Autodesk Inventor part; units mm, degrees
ref_plane "YZ Plane" through (0, 0, 0) normal (1, 0, 0) x (0, 1, 0)
ref_plane "XZ Plane" through (0, 0, 0) normal (0, 1, 0) x (-1, 0, 0)
ref_plane "XY Plane" through (0, 0, 0) normal (0, 0, 1) x (1, 0, 0)
sketch "Sketch1" plane through (0, 0, 0) normal (0, 0, 1) x (1, 0, 0)
  arc A0 (14.2748, -15.875) -> (15.875, -14.2748) centre (14.2748, -14.2748) ccw
  line L0 (15.875, -14.2748) -> (15.875, 14.2748)
  arc A1 (15.875, 14.2748) -> (14.2748, 15.875) centre (14.2748, 14.2748) ccw
  arc A2 (-14.2748, 15.875) -> (-15.875, 14.2748) centre (-14.2748, 14.2748) ccw
  line L1 (-15.875, 14.2748) -> (-15.875, -14.2748)
  arc A3 (-15.875, -14.2748) -> (-14.2748, -15.875) centre (-14.2748, -14.2748) ccw
  line L2 (-14.2748, -15.875) -> (14.2748, -15.875)
  line L3 (14.2748, 15.875) -> (-14.2748, 15.875)
  line L4 (-15.875, -19.05) -> (56.769, -19.05)
  line L5 (56.769, -19.05) -> (57.15, -18.669)
  line L6 (57.15, -18.669) -> (57.15, -16.256)
  line L7 (57.15, -16.256) -> (56.769, -15.875)
  line L8 (56.769, -15.875) -> (20.6502, -15.875)
  arc A4 (19.05, -14.2748) -> (20.6502, -15.875) centre (20.6502, -14.2748) ccw
  line L9 (19.05, -14.2748) -> (19.05, 15.875)
  arc A5 (19.05, 15.875) -> (15.875, 19.05) centre (15.875, 15.875) ccw
  line L10 (15.875, 19.05) -> (-15.875, 19.05)
  arc A6 (-15.875, 19.05) -> (-19.05, 15.875) centre (-15.875, 15.875) ccw
  line L11 (-19.05, 15.875) -> (-19.05, -15.875)
  arc A7 (-19.05, -15.875) -> (-15.875, -19.05) centre (-15.875, -15.875) ccw
  point P0 (0, 0)
extrude "Extrusion1" add sketch "Sketch1" against normal blind 304.8
hole "Hole1" at (0, 19.05, -19.05) direction (0, -1, 0) diameter 8.3312 end through all
hole "Hole2" at (-19.05, 0, -19.05) direction (1, 0, 0) diameter 8.3312 end through all
pattern_linear "Rectangular Pattern1" count 200 spacing 38.1 along (0, 0, -1) of "Hole1", "Hole2"
properties part number "9706"
Verification items for the finished model (mm, model axes). A direction names the side the tool comes from. Give positions to 0.01 mm unless a question says otherwise; leave off trailing zeros. Order: outer loops, then holes, each group sorted by start corner. A loop starts at its lowest first (then second) coordinate and runs counter-clockwise, first axis right, second up. Notation, with made-up numbers: M 10.25,-28 L 57.25,-28 A33 cw 57.25,5 Z; hole C 34,37 d8. An arc over 180 degrees is marked long. Return JSON: item names as keys, results as strings. Group by question number.
1) Go/stop test with flat-tipped pins: pin 1 Ø13.5 at (y, z) = (0, -133.35) entering from +X; pin 2 Ø11 at (x, z) = (36.5, -80) entering from +Y (3 decimals); pin 3 Ø6 at (x, z) = (20.5, -218) entering from +Y. Record where each tip stops, or that it passes through.
2) Scan lines: line 1 (X direction, y = -8, z = -247.5) (3 decimals); line 2 (Y direction, x = 17.65, z = -57.15). Record each from-to range of solid material in increasing order.
3) Section check A-A on x = -9. Record the cut outline in (y, z) (3 decimals), and give its area (3 significant figures).
4) Section check C-C on z = -209.55. Give the number of separate pieces and of enclosed holes in the cut face, and give its area (3 significant figures).
5) Section check B-B on z = -146. Record the cut outline in (x, y) (3 decimals), and give its area (3 significant figures).
6) Access from +Z, -Z, +X, -X, +Y, -Y to the whole of each face (thin tool, end or side, straight path). Record for faces 4 (the face through (0, -15.875, -150)), 5 (the face through (1.595, -17.485, -129.502)).
7) Mould release check, pull along X, two halves, no side actions. Record for faces 1 (the face through (16.05, -4.14, 0)), 2 (the face through (-15.875, 0, -150)), 3 (the face through (-0.18, 17.44, -175.61)): pulls with the +X half, pulls with the -X half, needs draft (parallel to the pull), parting line crosses it, or undercut.
Answer block:
{
 "1": {"pin 1": "stops at x = 19.05", "pin 2": "stops at y = -15.875", "pin 3": "stops at y = 18.6"},
 "2": {"line 1": "x = -19.05 to -15.875, 15.875 to 19.05", "line 2": "y = -19.05 to -4.17, 4.17 to 18.51"},
 "3": {"outline": "M -19.05,-304.8 L -15.875,-304.8 L -15.875,0 L -19.05,0 Z; M 15.875,-304.8 L 19.05,-304.8 L 19.05,0 L 15.875,0 Z", "area": "1,940 mm^2"},
 "4": {"separate pieces": "4", "enclosed holes": "0", "area": "455 mm^2"},
 "5": {"outline": "M -19.05,-15.875 A3.175 ccw -15.875,-19.05 L 56.769,-19.05 L 57.15,-18.669 L 57.15,-16.256 L 56.769,-15.875 L 20.65,-15.875 A1.6 cw 19.05,-14.275 L 19.05,15.875 A3.175 ccw 15.875,19.05 L -15.875,19.05 A3.175 ccw -19.05,15.875 Z; hole M -15.875,-14.275 A1.6 ccw -14.275,-15.875 L 14.275,-15.875 A1.6 ccw 15.875,-14.275 L 15.875,14.275 A1.6 ccw 14.275,15.875 L -14.275,15.875 A1.6 ccw -15.875,14.275 Z", "area": "561 mm^2"},
 "6": {"face 4": "+Z, -Z", "face 5": "+Y, -Y"},
 "7": {"face 1": "needs draft", "face 2": "undercut", "face 3": "undercut"}
}
